Input: part model. Units: mm. Frame: model coordinates. A direction names the side the tool comes from. Coordinates: 2 decimals unless noted, no trailing zeros. Order: outer loops, then holes, each group sorted by start corner. A loop starts at its lowest first (then second) coordinate and runs counter-clockwise, first axis right, second up. Notation, with made-up numbers: (-27.5, -7.5) -> (13.5, -7.5) arc R15 ccw to (13.5, 21.5) -> close; hole circle Ø11 at (33, -13.5). An arc over 180 degrees is marked (long way). Use one line per item in the form item = value. Start each with the question number.
1) Section query B-B on y = 36.9. Output: boundary loops of the cut face in (x, z) (3 decimals).
2) Pin query (flat end, axial travel): pin 1 (1 mm diameter, centred on y = 3, z = 2, fed in from +X). Return the tip coordinate at first contact, or that it passes through.
3) Section query A-A on x = 5.65. Output: boundary loops of the cut face in (y, z) (3 decimals).
4) Section query C-C on z = 0.5. Output: boundary loops of the cut face in (x, y).
5) Draft query along X for faces 1 (the flat face through (-3.8, 26, 2)), 2 (the flat face through (44, 8.95, 2)), 3 (the cylindrical face through (5.448, 38.437, 1.565)). Return one class per face: pulls with the +X half, pulls with the -X half, needs draft (parallel to the pull), parting line crosses it, or undercut.
6) Access query for faces 4 (the flat face through (42.3, 4, 2)), 5 (the flat face through (0, 5, 2)), 6 (the cylindrical face through (36.448, 38.437, 1.565)). Directions: +Z, -Z, +X, -X, +Y, -Y. A direction counts if a zero-diameter tool reaches every point of the face in a straight line with its end or side. Return the directions, or none.
7) Section query D-D on x = 21.15. Output: boundary loops of the cut face in (y, z) (3 decimals).
8) Ray query, line 1 along X through (y, z) = (37, 2.4); line 2 along Y through (x, z) = (5.65, 1.2); line 3 along Y through (x, z) = (21.15, 1). Return the intervals inside material, ascending.
from build123d import *

# Parameters (mm, degrees)
SKETCH1_R           = 11
SKETCH1_R_2         = 1.55
BOSS_EXTRUDE1_DEPTH = 3.175


with BuildPart() as part:
    # Sketch1 → Boss-Extrude1 (new body)
    with BuildSketch(Plane.XY):
        Polygon((0, 0), (42.3, 0), (42.3, 8.950102459), (46.1, 8.950102459), (46.1, 42.3), (42.3, 42.3), (0, 42.3), (-3.8, 42.3), (-3.8, 8.950102459), (0, 8.950102459), align=None)
        with Locations((21.15, 21.15)):
            Circle(SKETCH1_R, mode=Mode.SUBTRACT)
        with Locations((36.65, 36.9)):
            Circle(SKETCH1_R_2, mode=Mode.SUBTRACT)
        with Locations((5.65, 36.9)):
            Circle(SKETCH1_R_2, mode=Mode.SUBTRACT)
    extrude(amount=BOSS_EXTRUDE1_DEPTH)


solid = part.part
Answers below:
q1.outline = (-3.8, 0) -> (4.1, 0) -> (4.1, 3.175) -> (-3.8, 3.175) -> close; (7.2, 0) -> (35.1, 0) -> (35.1, 3.175) -> (7.2, 3.175) -> close; (38.2, 0) -> (46.1, 0) -> (46.1, 3.175) -> (38.2, 3.175) -> close
q2.pin_1 = 42.3
q3.outline = (0, 0) -> (35.35, 0) -> (35.35, 3.175) -> (0, 3.175) -> close; (38.45, 0) -> (42.3, 0) -> (42.3, 3.175) -> (38.45, 3.175) -> close
q4.outline = (-3.8, 8.95) -> (0, 8.95) -> (0, 0) -> (42.3, 0) -> (42.3, 8.95) -> (46.1, 8.95) -> (46.1, 42.3) -> (-3.8, 42.3) -> close; hole circle Ø3.1 at (5.65, 36.9); hole circle Ø22 at (21.15, 21.15); hole circle Ø3.1 at (36.65, 36.9)
q5.face_1 = pulls with the -X half
q5.face_2 = needs draft
q5.face_3 = undercut
q6.face_4 = +Z, -Z, +X, -Y
q6.face_5 = +Z, -Z, -X, -Y
q6.face_6 = +Z, -Z
q7.outline = (0, 0) -> (10.15, 0) -> (10.15, 3.175) -> (0, 3.175) -> close; (32.15, 0) -> (42.3, 0) -> (42.3, 3.175) -> (32.15, 3.175) -> close
q8.line_1 = -3.8 to 4.1, 7.2 to 35.1, 38.2 to 46.1
q8.line_2 = 0 to 35.35, 38.45 to 42.3
q8.line_3 = 0 to 10.15, 32.15 to 42.3
